The listing builds one solid part. Answer for the finished solid, in the listing's coordinates (mm). Face numbers are marked on the shaded views. A direction names the side the tool comes from. Coordinates: 2 decimals unless noted, no trailing zeros. Order: outer loops, then holes, each group sorted by start corner. A loop starts at its lowest first (then second) coordinate and runs counter-clockwise, first axis right, second up. Notation, with made-up numbers: (55, 45) -> (97, 45) arc R13 cw to (97, 53) -> close; hole circle Ø2 at (-23.5, 9). An arc over 180 degrees is marked (long way). Return JSON: item names as keys, results as strings.
from build123d import *

# Parameters (mm, degrees)
CHANFREIN2_SIZE    = 0.65
BOSS_EXTRU_1_REACH = 20.094
ESQUISSE3_R        = 2.43636475


with BuildPart() as part:
    # Esquisse1 → Révolution1 (revolve)
    with BuildSketch(Plane(origin=(0, 0, 0), x_dir=(0, 0, -1), z_dir=(1, 0, 0)), mode=Mode.PRIVATE) as r_volution1_sk:
        with BuildLine():
            Line((17.5, 2), (2.8, 2))
            Line((2.8, 2), (2.8, 3.25))
            Line((2.8, 3.25), (2.07, 3.25))
            ThreePointArc((2.07, 3.25), (0.957918357, 3.039288677), (0, 2.43636475))
            Line((0, 2.43636475), (0, 0))
            Line((0, 0), (17.5, 0))
            Line((17.5, 0), (17.5, 2))
        make_face()
    revolve(r_volution1_sk.sketch.rotate(Axis((0, 0, -17.5), (0, 0, -1)), 90), axis=Axis((0, 0, -17.5), (0, 0, -1)))

    # Chanfrein2
    chanfrein2_edges = [part.edges().sort_by_distance(p)[0] for p in [
        (-2, 0, -17.5),
    ]]
    chamfer(chanfrein2_edges, length=CHANFREIN2_SIZE)

    # Esquisse2 → Enlèvement de matière-Révolution1 (revolve, cut)
    with BuildSketch(Plane(origin=(0, 0, 0), x_dir=(0, 0, -1), z_dir=(1, 0, 0)), mode=Mode.PRIVATE) as enl_vement_de_mati_re_r_volution1_sk:
        Polygon((0, 0), (0, 2.049593456), (2, 2.049593456), (3.183333333, 0), align=None)
    revolve(enl_vement_de_mati_re_r_volution1_sk.sketch.rotate(Axis((0, 0, 0), (0, 0, -1)), 90), axis=Axis((0, 0, 0), (0, 0, -1)), mode=Mode.SUBTRACT)

    # Boss.-Extru.1: up to this cone (the profile starts inside it)
    boss_extru_1_end = Plane(origin=(0, 0, 0), z_dir=(0, 0, 1)).offset(-3.183332333) * Cone(1.732e-06, 50.733549402, 29.291027404, align=(Align.CENTER, Align.CENTER, Align.MIN), mode=Mode.PRIVATE)
    # Esquisse3 → Boss.-Extru.1 (add, up to the surface)
    with BuildSketch(Plane.XY, mode=Mode.PRIVATE) as boss_extru_1_sk1:
        Circle(ESQUISSE3_R)
        Polygon((0, 2.049593456), (-1.775, 1.024796728), (-1.775, -1.024796728), (0, -2.049593456), (1.775, -1.024796728), (1.775, 1.024796728), align=None, mode=Mode.SUBTRACT)
    boss_extru_1_tool1 = extrude(boss_extru_1_sk1.sketch, amount=-BOSS_EXTRU_1_REACH, mode=Mode.PRIVATE) & boss_extru_1_end
    add(boss_extru_1_tool1.solids().sort_by_distance((-2.367454, 0, 0))[0])


solid = part.part
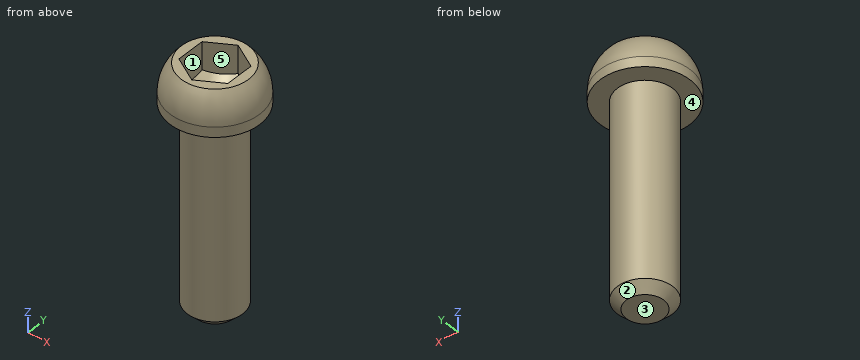
1. The part is cut by section A-A on z = -10.5. Give the vertices of the cut face in (x, y), and give its area (3 significant figures).
Answer block:
{"outline": "circle Ø4 at (0, 0)", "area": "12.6 mm2"}
2. For the marked faces 4 and 5, determine the directions among +Z, -Z, +X, -X, +Y, -Y from which every point of the face is accessible in a straight line to the end or side of a thin tool.
Answer block:
{"face 4": "-Z", "face 5": "+Z"}
3. The part is cut by section B-B on z = -3. Give the vertices of the cut face in (x, y).
Answer block:
{"outline": "circle Ø4 at (0, 0); hole circle Ø0.64 at (0, 0)"}
4. Determine the mould class of the marked faces 1, 2 and 3 for opening direction Y: pulls with the +Y half, pulls with the -Y half, needs draft (parallel to the pull), parting line crosses it, or undercut.
Answer block:
{"face 1": "undercut", "face 2": "parting line crosses it", "face 3": "needs draft"}
5. Each of these flat-tipped pins is pushed along its axis until it touches: pin 1 Ø3 at (x, z) = (-0.5, -13) entering from +Y; pin 2 Ø2.5 at (y, z) = (0.5, -1.5) entering from -X; pin 3 Ø1 at (x, z) = (-2, -14) entering from -Y; pin 4 Ø1 at (y, z) = (0.5, -1) entering from +X. Where does it stop, or does it pass through?
Answer block:
{"pin 1": "stops at y = 2", "pin 2": "stops at x = -3.25", "pin 3": "stops at y = -1.32", "pin 4": "stops at x = 3.17"}
6. Consider line 1 (Z direction, x = 0.5, y = 2.25); line 2 (Y direction, x = 2.5, z = -1.75); line 3 (Y direction, x = 1.5, z = -15.5). Determine where each line is inside the solid, lowest interval first. Write a range as from..to.
Answer block:
{"line 1": "z = -2.8..0", "line 2": "y = -2.05..2.05", "line 3": "y = -1.32..1.32"}
